```python
from build123d import *

# Parameters (mm, degrees)
SKETCH2_R                = 12.25
SKETCH2_R_2              = 9.25
BOSS_EXTRUDE1_DEPTH      = 210
SKETCH5_R                = 9.5
SKETCH5_R_2              = 4.625
BOSS_EXTRUDE2_DEPTH      = 12
BOSS_EXTRUDE3_DEPTH      = 1
CIRPATTERN1_COUNT        = 3
SKETCH8_R                = 4
SKETCH8_R_2              = 2.5
BOSS_EXTRUDE4_DEPTH      = 6.35
BOSS_EXTRUDE4_DEPTH_BACK = 6.35
SKETCH9_W                = 2
SKETCH9_H                = 19.5


with BuildPart() as part:
    # Sketch2 → Boss-Extrude1 (new body)
    with BuildSketch(Plane(origin=(-2.465768249, 0, -0.081027564), x_dir=(1, 0, 0), z_dir=(0, 1, 0))):
        with Locations((2.411661176, 0)):
            Circle(SKETCH2_R)
        with Locations((2.411661176, 0)):
            Circle(SKETCH2_R_2, mode=Mode.SUBTRACT)
    extrude(amount=BOSS_EXTRUDE1_DEPTH)

    # Sketch5 → Boss-Extrude2 (add)
    with BuildSketch(Plane(origin=(0, 60, 0), x_dir=(1, 0, 0), z_dir=(0, 1, 0))):
        with Locations((-0.054107074, 0.081027564)):
            Circle(SKETCH5_R)
        with Locations((-0.054107074, 0.081027564)):
            Circle(SKETCH5_R_2, mode=Mode.SUBTRACT)
    extrude(amount=BOSS_EXTRUDE2_DEPTH)

    # Sketch7 → Boss-Extrude3 (add, symmetric)
    with BuildSketch(Plane.XY):
        Polygon((12.195892926, 75.2), (9.828211369, 75.2), (11.195892926, 0), (12.195892926, 0), (37.059460314, -30), (45.34731611, -30), (45.34731611, 9), align=None)
    boss_extrude3 = extrude(amount=BOSS_EXTRUDE3_DEPTH, both=True)

    # CirPattern1: Boss-Extrude3 ×3 about axis
    cirpattern1_axis = Axis((-0.054107074, 0, -0.081027564), (0, 1, 0))
    for i in range(1, CIRPATTERN1_COUNT):
        add(boss_extrude3.rotate(cirpattern1_axis, i * 360 / CIRPATTERN1_COUNT))

    # Sketch8 → Boss-Extrude4 (add, two sides)
    with BuildSketch(Plane(origin=(0.379836366, 95, 0), x_dir=(1, 0, 0), z_dir=(0, 1, 0))) as boss_extrude4_sk:
        with Locations((-15.3, 0)):
            Circle(SKETCH8_R)
        with Locations((-15.3, 0)):
            Circle(SKETCH8_R_2, mode=Mode.SUBTRACT)
    extrude(amount=BOSS_EXTRUDE4_DEPTH)
    extrude(boss_extrude4_sk.sketch, amount=-BOSS_EXTRUDE4_DEPTH_BACK)

    # Sketch9 → Revolve-Thin1 (revolve)
    with BuildSketch(Plane(origin=(0, 110, 0), x_dir=(1, 0, 0), z_dir=(0, 1, 0))):
        with Locations((-2.5, 0.25)):
            Rectangle(SKETCH9_W, SKETCH9_H)
    revolve(axis=Axis((-3.5, 110, -10), (0, 0, 1)))


solid = part.part
```
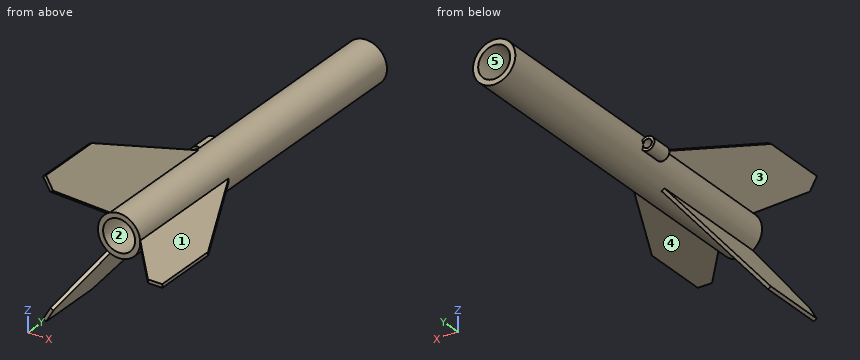
Here's how the part is built. I have some questions about the finished solid (model axes, mm). Face numbers are marked on the shaded views. A direction names the side the tool comes from. Give positions to 0.01 mm unless a question says otherwise; leave off trailing zeros. Order: outer loops, then holes, each group sorted by start corner. A loop starts at its lowest first (then second) coordinate and runs counter-clockwise, first axis right, second up. Notation, with made-up numbers: (10.5, -13.75) -> (32.5, -13.75) arc R15 cw to (32.5, 12.25) -> close; hole circle Ø8 at (83.25, 83.25). An arc over 180 degrees is marked (long way). Use CSV: the item, a comma, the result in double quotes. Start each with the question number.
Item 1: If I drill on probe 1 along Z at (x, y) = (35.5, 11.5); probe 2 along Z at (x, y) = (-3.5, 90.5); probe 3 along Z at (x, y) = (5.5, 137.5), over which ranges is the centre line in solid material (lowest first)? Write a range as [from, to].
Item 2: Suppose I cut it at A-A (y = 193). List the corners of the cut face in (x, z) for me, and give its area (3 significant figures).
Item 3: Suppose I cut it at B-B (z = 27). List the corners of the cut face in (x, y) for me.
Item 4: Suppose I cut it at D-D (z = -22.5). List the corners of the cut face in (x, y) for me.
Item 5: I'm going to push flat-ended pins straight in: P1, Ø10, axis at x = 34, y = 26.5, coming from the +Z side; P2, Ø2, axis at y = 123.5, z = 13.5, coming from the +X side; P3, Ø6, axis at y = 34, z = 9, coming from the -X side; P4, Ø9, axis at x = 0, z = -2, coming from the +Y side. Where does each tip first touch, or does it pass through?
Item 6: On a 3-axis mill with a long thin cutter (end or side, diameter ignored), from which of +Z, -Z, +X, -X, +Y, -Y can I reach the whole of each face in a straight line? I mean the marked faces 1 and 2. Say none if no direction works.
Item 7: Suppose I cut it at C-C (y = 34). List the corners of the cut face in (x, z) for me.
Item 8: Thinking about a two-plate mould opening in X: for the marked faces 3, 4 and 5, which applies, pulls with the +X half, pulls with the -X half, needs draft (parallel to the pull), parting line crosses it, or undercut?
Answer block:
1,probe 1,"z = [-1, 1]"
1,probe 2,"z = [-11.84, -8.67], [8.5, 11.67]"
1,probe 3,"z = [-11, -7.48], [7.32, 10.84]"
2,outline,"circle Ø24.5 at (-0.05, -0.08); hole circle Ø18.5 at (-0.05, -0.08)"
2,area,"203 mm^2"
3,outline,"(-16.94, -23.7) -> (-14.63, -22.31) -> (-14.63, 38.28) -> (-16.94, 35.97) -> close"
4,outline,"(-14.06, -17.09) -> (-11.75, -15.7) -> (-11.75, 49.21) -> (-14.06, 46.91) -> close"
5,P1,"stops at z = 1"
5,P2,"passes through"
5,P3,"stops at x = -10.69"
5,P4,"stops at y = 112"
6,face 1,"+Z, +X, +Y, -Y"
6,face 2,"-Y"
7,outline,"(-17.43, 27.86) -> (-7.09, 9.95) arc R12.25 ccw to (-6.96, -10.2) -> (-17.29, -28.1) -> (-15.56, -29.1) -> (-5.22, -11.19) arc R12.25 ccw to (12.16, -1) -> (32.83, -1) -> (32.83, 1) -> (12.15, 1) arc R12.25 ccw to (-5.37, 10.96) -> (-15.7, 28.86) -> close; hole circle Ø18.5 at (-0.05, -0.08)"
8,face 3,"pulls with the -X half"
8,face 4,"needs draft"
8,face 5,"undercut"
